```python
from build123d import *

# Parameters (mm, degrees)
SKETCH4_R          = 4.75
SKETCH3_R          = 4.25
SKETCH7_R          = 5
CUT_EXTRUDE4_DEPTH = 3
SKETCH8_R          = 3
CUT_EXTRUDE5_DEPTH = 2.5
CUT_EXTRUDE6_DEPTH = 7


with BuildPart() as part:
    # Sketch2 → Revolve1 (revolve)
    with BuildSketch(Plane.XY):
        with BuildLine():
            Line((0, 0), (32.5, 0))
            ThreePointArc((32.5, 0), (16.25, 16.25), (0, 0))
        make_face()
    revolve(axis=Axis((0, 0, 0), (1, 0, 0)))

    # Sketch4 → Cut-Loft1 section 0
    with BuildSketch(Plane(origin=(0, 0, 0), x_dir=(1, 0, 0), z_dir=(0, 1, 0))):
        with Locations((16.25, 0)):
            Circle(SKETCH4_R)
    # Sketch3 → Cut-Loft1 section 1
    with BuildSketch(Plane(origin=(0, 16.25, 0), x_dir=(1, 0, 0), z_dir=(0, 1, 0))):
        with Locations((16.25, 0)):
            Circle(SKETCH3_R)
    loft(mode=Mode.SUBTRACT)

    # Sketch7 → Cut-Extrude4 (cut)
    with BuildSketch(Plane(origin=(0, -17, 0), x_dir=(1, 0, 0), z_dir=(0, 1, 0))):
        with Locations((16.25, 0)):
            Circle(SKETCH7_R)
    extrude(amount=CUT_EXTRUDE4_DEPTH, mode=Mode.SUBTRACT)

    # Sketch8 → Cut-Extrude5 (cut)
    with BuildSketch(Plane.XZ.offset(14)):
        with Locations((16.25, 0)):
            Circle(SKETCH8_R)
    extrude(amount=-CUT_EXTRUDE5_DEPTH, mode=Mode.SUBTRACT)

    # Sketch9 → Cut-Extrude6 (cut)
    with BuildSketch(Plane.XZ.offset(11.5)):
        with BuildLine():
            Line((14.25, 2.236067977), (14.25, -2.236067977))
            ThreePointArc((14.25, -2.236067977), (16.25, -3), (18.25, -2.236067977))
            Line((18.25, -2.236067977), (18.25, 2.236067977))
            ThreePointArc((18.25, 2.236067977), (16.25, 3), (14.25, 2.236067977))
        make_face()
    extrude(amount=-CUT_EXTRUDE6_DEPTH, mode=Mode.SUBTRACT)


solid = part.part
```
For this review, take the finished solid that the model builds, in its own axes (mm). A direction names the side the tool comes from. Give positions to 0.01 mm unless a question says otherwise; leave off trailing zeros. Write each loop counter-clockwise with the first axis right and the second up, starting at its lowest first coordinate (ties: lowest second). Pieces come first, ordered by that corner, then holes.
Item 1: Take a section at B-B (y = -11). Give the boundary of the cut face in (x, z).
Item 2: Machinability: for faces 1 (the face through (18.25, -8, 0)), 2 (the face through (16, 0, 0)), which of the approach directions +Z, -Z, +X, -X, +Y, -Y give a long, thin tool a straight path to every point of the face, cutting with its end or side? Answer none if there is none.
Item 3: Insertion check: P1, Ø1.1, axis at x = 13.5, z = 1, coming from the -Y side; P2, Ø12, axis at y = -3.5, z = -7.5, coming from the -X side; P3, Ø1.3, axis at y = -9.5, z = -1, coming from the -X side. Each pin has a flat end and moves straight along its axis. Give the tip position at first contact, or say it passes through.
Item 4: Take a section at C-C (z = 6.5). Give the boundary of the cut face in (x, y).
Item 5: Wall thickness on probe 1 along Z at (x, y) = (16.25, -14.4); probe 2 along X at (y, z) = (7.5, 0); probe 3 along X at (y, z) = (-13, 0): over which ranges is each line inside the solid? List them lowest first.
Item 6: Take a section at A-A (x = 16.25). Give the boundary of the cut face in (y, z), and give its area (3 significant figures).
Item 7: Take a section at D-D (x = 8). Give the boundary of the cut face in (y, z), and give its area (3 significant figures).
Established:
1. outline: circle Ø23.92 at (16.25, 0); hole (14.25, -2.24) arc R3 ccw to (18.25, -2.24) - (18.25, 2.24) arc R3 ccw to (14.25, 2.24) - close
2. face 1: -Y
2. face 2: none
3. P1: stops at y = -14
3. P2: stops at x = 0.16
3. P3: stops at x = 2.66
4. outline: circle Ø29.79 at (16.25, 0)
5. probe 1: z = -7.53 to -5, 5 to 7.53
5. probe 2: x = 1.83 to 11.73, 20.77 to 30.67
5. probe 3: x = 6.5 to 13.25, 19.25 to 26
6. outline: (-15.46, -5) arc R16.25 ccw to (15.68, -4.27) - (0, -4.75) - (0, 4.75) - (15.68, 4.27) arc R16.25 ccw to (-15.46, 5) - (-14, 5) - (-14, 3) - (-4.5, 3) - (-4.5, -3) - (-14, -3) - (-14, -5) - close
6. area: 608 mm2
7. outline: circle Ø28 at (0, 0)
7. area: 616 mm2
